Source: CAD feature listing. Evaluate the final solid. Frame: model axes, mm. Face numbers are marked on the shaded views. A direction names the side the tool comes from. Coordinates: 2 decimals unless noted, no trailing zeros. Order: outer loops, then holes, each group sorted by start corner. A loop starts at its lowest first (then second) coordinate and runs counter-clockwise, first axis right, second up.
```python
from build123d import *

# Parameters (mm, degrees)
F1_DEPTH = 63.5
F0_W     = 28.067
F0_H     = 19.05
F2_DEPTH = 25.4
F3_DEPTH = 3.175


with BuildPart() as f1:
    # F0 (on Front) → F1 (new body, symmetric)
    with BuildSketch(Plane.XZ):
        Polygon((-41.275, 9.525), (-41.275, -9.525), (41.275, -9.525), (41.275, 9.525), (22.225, 9.525), align=None)
    extrude(amount=F1_DEPTH, both=True)

    # F0 (on Front) → F2 (join, symmetric)
    with BuildSketch(Plane.XZ):
        with BuildLine():
            Line((22.225, 9.525), (41.275, 9.525))
            Line((41.275, 9.525), (41.275, 53.5730462312))
            ThreePointArc((41.275, 53.5730462312), (45.9246798487, 64.7983663825), (57.15, 69.4480462312))
            Line((57.15, 69.4480462312), (66.675, 69.4480462312))
            Line((66.675, 69.4480462312), (66.675, 88.4980462312))
            Line((66.675, 88.4980462312), (57.15, 88.4980462312))
            add(Edge.make_bspline(
                [(55.0500442631, 88.4348564381), (55.7636307959, 88.4570758509), (56.4639128881, 88.477925733), (57.15, 88.4980462312)],
                knots=[123.5650142277, 123.5650142277, 123.5650142277, 123.5650142277, 126.1912146547, 126.1912146547, 126.1912146547, 126.1912146547], degree=3))
            ThreePointArc((55.0500442631, 88.4348564381), (31.7226861514, 77.5147950279), (22.225, 53.5730462312))
            Line((22.225, 53.5730462312), (22.225, 9.525))
        make_face()
        with Locations((80.7085, 78.9730462312)):
            Rectangle(F0_W, F0_H)
    extrude(amount=F2_DEPTH, both=True)

    # F0 (on Front) → F3 (join, symmetric)
    with BuildSketch(Plane.XZ):
        with BuildLine():
            add(Edge.make_bspline(
                [(-41.275, 9.525), (-41.5528520698, 83.3121254449), (21.4751772531, 87.3894137404), (55.0500442631, 88.4348564381)],
                knots=[0, 0, 0, 0, 123.5650142277, 123.5650142277, 123.5650142277, 123.5650142277], degree=3))
            Line((-41.275, 9.525), (22.225, 9.525))
            Line((22.225, 9.525), (22.225, 53.5730462312))
            ThreePointArc((22.225, 53.5730462312), (31.7226861514, 77.5147950279), (55.0500442631, 88.4348564381))
        make_face()
    extrude(amount=F3_DEPTH, both=True)

    # F0 (on Front) → F4 (revolve)
    with BuildSketch(Plane.XZ):
        Polygon((94.742, 93.6625), (94.742, 88.4980462312), (94.742, 69.4480462312), (94.742, 65.0875), (117.475, 65.0875), (117.475, 93.6625), align=None)
    revolve(axis=Axis((94.742, 0, 79.375), (0, 0, 1)))


solid = f1.part
```
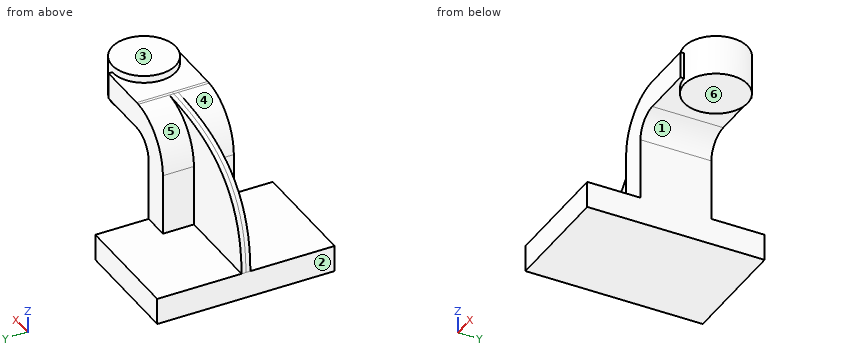
1. Section query B-B on y = -44.5. Return loops of the section in (x, z) (3 decimals).
Findings:
outline: (-41.275, -9.525) - (41.275, -9.525) - (41.275, 9.525) - (-41.275, 9.525) - close
2. Draft query along X for the marked faces 1, 2 and 3. Return one class per face: released by +X, released by -X, zero draft, split by the parting line, or undercut.
Findings:
face 1: undercut
face 2: released by -X
face 3: zero draft
3. Section query A-A on z = -0.5. Return loops of the section in (x, y) (3 decimals), plus the area to 3 significant figures.
Findings:
outline: (-41.275, -63.5) - (41.275, -63.5) - (41.275, 63.5) - (-41.275, 63.5) - close
area: 10,500 mm2
4. Pin query (flat end, axial travel): P1, Ø1, axis at x = -9, z = 16.5, coming from the -Y side (3 decimals); P2, Ø4, axis at x = 43, z = 60, coming from the -Y side; P3, Ø1.5, axis at y = -0.5, z = 70, coming from the -X side. Return the tip coordinate at first contact, or that it passes through.
Findings:
P1: stops at y = -3.175
P2: stops at y = -25.4
P3: stops at x = -16.69
5. Ray query, line 1 (Z direction, x = -18.5, y = 11.5) (3 decimals); line 2 (Y direction, x = 5, z = 65) (3 decimals); line 3 (X direction, y = -22, z = 3) (3 decimals). Return the intervals inside material, ascending.
Findings:
line 1: z = -9.525 to 9.525
line 2: y = -3.175 to 3.175
line 3: x = -41.275 to 41.275
6. Access query for the marked faces 4, 5 and 6. Directions: +Z, -Z, +X, -X, +Y, -Y. A direction counts if a zero-diameter tool reaches every point of the face in a straight line with its end or side. Return the directions, or none.
Findings:
face 4: +Z, -X, -Y
face 5: +Z, -X, +Y
face 6: -Z, +X, +Y, -Y
